Print and shaded views of the part. All mm, measured from the part's lowest x, y and z. Round coordinates to 2 decimals unless told otherwise and drop trailing zeros. Loops run counter-clockwise (first coordinate to the right, second up) from the corner with the lowest first, then second, coordinate; pieces in that order, holes last. Notation, with made-up numbers: (48, 14) - (72, 14) arc R29 ccw to (72, 45) - close; hole circle Ø8 at (9, -10.75). An arc over 180 degrees is marked (long way). Use one line per item in the form item = value.
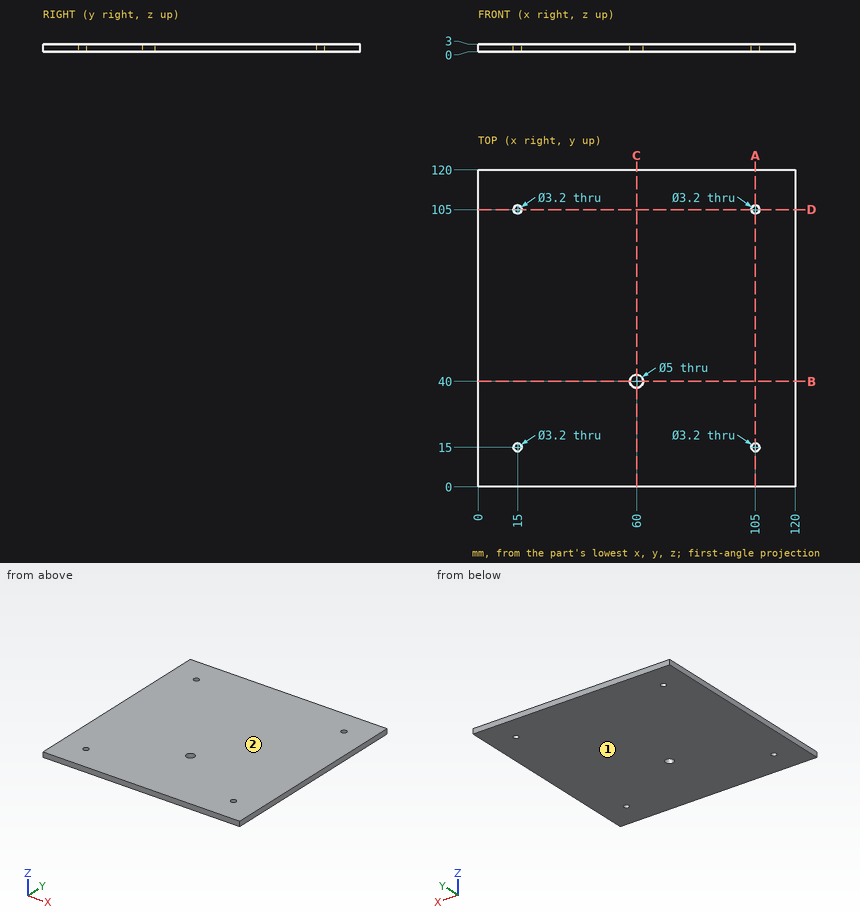
1) Flat gauge pin, fed straight in: pin 1 (1.5 mm diameter, centred on y = 81.5, z = 0.5, fed in from -X). Where does the tip first touch, or does it go through?
Report:
pin_1 = 0
2) Two-plate mould, pull along Z, no slides. Class the marked faces 1 and 2: +Z half, -Z half, draft (parallel to the pull), parting line (faces both ways), or undercut.
Report:
face_1 = -Z half
face_2 = +Z half
3) Slice it at C-C (x = 60). Write the cut outline in (y, z).
Report:
outline = (0, 0) - (37.5, 0) - (37.5, 3) - (0, 3) - close; (42.5, 0) - (120, 0) - (120, 3) - (42.5, 3) - close
4) Slice it at A-A (x = 105). Write the cut outline in (y, z), plus the area to 3 significant figures.
Report:
outline = (0, 0) - (13.4, 0) - (13.4, 3) - (0, 3) - close; (16.6, 0) - (103.4, 0) - (103.4, 3) - (16.6, 3) - close; (106.6, 0) - (120, 0) - (120, 3) - (106.6, 3) - close
area = 341 mm^2
5) Drill centre lines: probe 1 along Y at (x, z) = (105, 1.15); probe 2 along Y at (x, z) = (106, 1.5). Where is each one in solid material? Low to high.
Report:
probe_1 = 0 to 13.4, 16.6 to 103.4, 106.6 to 120
probe_2 = 0 to 13.75, 16.25 to 103.75, 106.25 to 120
6) Slice it at B-B (y = 40). Write the cut outline in (x, z), plus the area to 3 significant figures.
Report:
outline = (0, 0) - (57.5, 0) - (57.5, 3) - (0, 3) - close; (62.5, 0) - (120, 0) - (120, 3) - (62.5, 3) - close
area = 345 mm^2
